Geometry check sheet. Reference: the model listing, model coordinates, mm. A direction names the side the tool comes from. Coordinates: 2 decimals unless noted, no trailing zeros. Loops run counter-clockwise (first coordinate to the right, second up) from the corner with the lowest first, then second, coordinate; pieces in that order, holes last. Notation, with made-up numbers: (9, 5.25) -> (19, 5.25) arc R12 ccw to (19, 19.25) -> close; hole circle Ø10 at (-15.5, -10.5). An arc over 180 degrees is marked (long way). Answer as a JSON object with one key per item and string values.
from build123d import *

# Parameters (mm, degrees)
BOSS_EXTRU_1_DEPTH       = 8
REPOSE_MOTEUR_DEPTH      = 8
ESQUISSE5_R              = 8.25
FIXATION_COURROI_1_DEPTH = 6
ESQUISSE6_R              = 5.75
FIXATION_COURROI_2_DEPTH = 2
ESQUISSE3_R              = 7
FIXATION_MOTEUR_1_DEPTH  = 2
ESQUISSE2_R              = 13.25
FIXATION_MOTEUR_2_DEPTH  = 6
D_GAGEMENT_M31_D         = 3.2
D_GAGEMENT_M31_DEPTH     = 10
D_GAGEMENT_M31_TIP       = 0.96137699
D_GAGEMENT_M41_D         = 4.3
D_GAGEMENT_M41_DEPTH     = 10
D_GAGEMENT_M41_TIP       = 1.291850331
ESQUISSE7_R              = 1.75
ENL_V_MAT_EXTRU_1_DEPTH  = 10


with BuildPart() as part:
    # Esquisse1 → Boss.-Extru.1 (new body)
    with BuildSketch(Plane.XY):
        Polygon((-53.385579659, 37.671052632), (-53.385579659, -32.328947368), (72.614420341, -32.328947368), (72.614420341, 12.671052632), (-18.385579659, 12.671052632), (-18.385579659, 37.671052632), align=None)
    extrude(amount=BOSS_EXTRU_1_DEPTH)

    # Esquisse4 → Repose moteur (cut)
    with BuildSketch(Plane.XY.offset(8)):
        with BuildLine():
            Line((42.741726231, 12.671052632), (67.614420341, 12.671052632))
            ThreePointArc((67.614420341, 12.671052632), (55.178073286, 4.423411332), (42.741726231, 12.671052632))
        make_face()
        with BuildLine():
            Line((-19.611662647, 7.796589582), (-33.760042708, -9.10286438))
            ThreePointArc((-33.760042708, -9.10286438), (-33.385579659, -13.328947368), (-29.15949667, -12.954484319))
            Line((-29.15949667, -12.954484319), (-15.011116609, 3.944969643))
            ThreePointArc((-15.011116609, 3.944969643), (-15.385579659, 8.171052632), (-19.611662647, 7.796589582))
        make_face()
    extrude(amount=-REPOSE_MOTEUR_DEPTH, mode=Mode.SUBTRACT)

    # Esquisse5 → Fixation courroi 1 (cut)
    with BuildSketch(Plane.XY.offset(8)):
        with Locations((9.364420341, -14.328947368)):
            Circle(ESQUISSE5_R)
    extrude(amount=-FIXATION_COURROI_1_DEPTH, mode=Mode.SUBTRACT)

    # Esquisse6 → Fixation courroi 2 (cut)
    with BuildSketch(Plane(origin=(0, 0, 0), x_dir=(-1, 0, 0), z_dir=(0, 0, -1))):
        with Locations((-9.364420341, -14.328947368)):
            Circle(ESQUISSE6_R)
    extrude(amount=-FIXATION_COURROI_2_DEPTH, mode=Mode.SUBTRACT)

    # Esquisse3 → Fixation moteur 1 (cut)
    with BuildSketch(Plane(origin=(0, 0, 0), x_dir=(-1, 0, 0), z_dir=(0, 0, -1))):
        with Locations((35.885579659, 17.671052632)):
            Circle(ESQUISSE3_R)
    extrude(amount=-FIXATION_MOTEUR_1_DEPTH, mode=Mode.SUBTRACT)

    # Esquisse2 → Fixation moteur 2 (cut)
    with BuildSketch(Plane.XY.offset(8)):
        with Locations((-36.135579659, 17.671052632)):
            Circle(ESQUISSE2_R)
    extrude(amount=-FIXATION_MOTEUR_2_DEPTH, mode=Mode.SUBTRACT)

    # Dégagement M31
    with Locations(Plane(origin=(-26.385579659, 17.671052632, 0), x_dir=(-1, 0, 0), z_dir=(0, 0, -1))):
        with Locations((0, 0), (9.5, 9.5), (19, 0), (9.5, -9.5)):
            Hole(D_GAGEMENT_M31_D / 2, depth=D_GAGEMENT_M31_DEPTH)
            with Locations((0, 0, -(D_GAGEMENT_M31_DEPTH + D_GAGEMENT_M31_TIP / 2))):  # 118° drill point
                Cone(0, D_GAGEMENT_M31_D / 2, D_GAGEMENT_M31_TIP, mode=Mode.SUBTRACT)

    # Dégagement M41
    with Locations(Plane(origin=(-10.635579659, 12.671052632, 4), x_dir=(1, 0, 0), z_dir=(0, 1, 0))):
        with Locations((0, 0), (40, 0)):
            Hole(D_GAGEMENT_M41_D / 2, depth=D_GAGEMENT_M41_DEPTH)
            with Locations((0, 0, -(D_GAGEMENT_M41_DEPTH + D_GAGEMENT_M41_TIP / 2))):  # 118° drill point
                Cone(0, D_GAGEMENT_M41_D / 2, D_GAGEMENT_M41_TIP, mode=Mode.SUBTRACT)

    # Esquisse7 → Enlèv. mat.-Extru.1 (cut)
    with BuildSketch(Plane.XZ.offset(32.328947368)):
        with Locations((-49.385579659, 3.800276617)):
            Circle(ESQUISSE7_R)
        with Locations((-14.385579659, 3.800276617)):
            Circle(ESQUISSE7_R)
        with Locations((37.614420341, 3.800276617)):
            Circle(ESQUISSE7_R)
        with Locations((68.614420341, 3.800276617)):
            Circle(ESQUISSE7_R)
    extrude(amount=-ENL_V_MAT_EXTRU_1_DEPTH, mode=Mode.SUBTRACT)


solid = part.part
1. Section check D-D, the plane x = 20. Record the boundary of the cut face in (y, z), then the cut area to 3 significant figures.
Evaluation:
{"outline": "(-32.33, 0) -> (12.67, 0) -> (12.67, 8) -> (-32.33, 8) -> close", "area": "360 mm^2"}
2. Section check B-B, the plane x = -45. Record the boundary of the cut face in (y, z), then the cut area to 3 significant figures.
Evaluation:
{"outline": "(-32.33, 0) -> (16.12, 0) -> (16.12, 2) -> (7.82, 2) -> (7.82, 8) -> (-32.33, 8) -> close; (19.22, 0) -> (37.67, 0) -> (37.67, 8) -> (27.52, 8) -> (27.52, 2) -> (19.22, 2) -> close", "area": "436 mm^2"}
3. Section check A-A, the plane y = -11. Record the boundary of the cut face in (x, z), then the cut area to 3 significant figures.
Evaluation:
{"outline": "(-53.39, 0) -> (-34.46, 0) -> (-34.46, 8) -> (-53.39, 8) -> close; (-27.52, 0) -> (4.68, 0) -> (4.68, 2) -> (1.82, 2) -> (1.82, 8) -> (-27.52, 8) -> close; (14.05, 0) -> (72.61, 0) -> (72.61, 8) -> (16.91, 8) -> (16.91, 2) -> (14.05, 2) -> close", "area": "843 mm^2"}
4. Section check C-C, the plane y = 14.5. Record the boundary of the cut face in (x, z), then the cut area to 3 significant figures.
Evaluation:
{"outline": "(-53.39, 0) -> (-42.13, 0) -> (-42.13, 2) -> (-49, 2) -> (-49, 8) -> (-53.39, 8) -> close; (-29.65, 0) -> (-18.39, 0) -> (-18.39, 8) -> (-23.27, 8) -> (-23.27, 2) -> (-29.65, 2) -> close", "area": "101 mm^2"}
5. Depth check by flat-ended pin: P1, Ø1.7, axis at x = 38, z = 3.5, coming from the -Y side; P2, Ø2.5, axis at x = 71, z = 4.5, coming from the +Y side. Enter the tip coordinate at first touch or a pass-through.
Evaluation:
{"P1": "stops at y = -22.33", "P2": "stops at y = 12.67"}
6. Mould release check, pull along Z, two halves, no side actions. Record for faces 1 (the face through (69, -22.329, 4)), 2 (the face through (3.7, -16, 2)), 3 (the face through (72.614, -10, 4)): released by +Z, released by -Z, zero draft, split by the parting line, or undercut.
Evaluation:
{"face 1": "undercut", "face 2": "released by +Z", "face 3": "zero draft"}
7. Tool access check on faces 4 (the face through (-23.896, 12.596, 5.042)), 5 (the face through (-12.716, -27.399, 4.326)), 6 (the face through (-26.587, -0.535, 4.056)), 7 (the face through (70, 12.671, 4)). Record the directions out of +Z, -Z, +X, -X, +Y, -Y that give a thin tool (end or side, any length) a straight path to the whole face; none if there is none.
Evaluation:
{"face 4": "+Z", "face 5": "-Y", "face 6": "+Z, -Z", "face 7": "+Z, -Z, +X, +Y"}
8. Thickness scan on probe 1 along Z at (x, y) = (-14.5, -25); probe 2 along Y at (x, z) = (-26.5, 1.5); probe 3 along Y at (x, z) = (-28.5, 6.25). Record the ranges inside material, lowest first. Write a range as from..to.
Evaluation:
{"probe 1": "z = 0..2.05, 5.55..8", "probe 2": "y = -32.33..-9.78, -0.43..16.08, 19.27..37.67", "probe 3": "y = -32.33..-12.17, -2.82..6.84, 28.5..37.67"}
